from build123d import *

# Parameters (mm, degrees)
BOSS_EXTRUDE1_DEPTH = 1.5875
SKETCH3_W           = 9.525
SKETCH3_H           = 2.54
CUT_EXTRUDE1_DEPTH  = 29.598819744
SKETCH4_R           = 1.5875
BOSS_EXTRUDE2_DEPTH = 2.54
BOSS_EXTRUDE3_DEPTH = 1.778
SKETCH6_W           = 48.787
SKETCH6_H           = 0.4318
CUT_EXTRUDE2_DEPTH  = 19.05


with BuildPart() as part:
    # Sketch2 → Boss-Extrude1 (new body)
    with BuildSketch(Plane.XY):
        with BuildLine():
            Line((21.2185, 2.909935566), (21.2185, 11.9225))
            ThreePointArc((21.2185, 11.9225), (20.362958908, 13.987958908), (18.2975, 14.8435))
            Line((18.2975, 14.8435), (-18.2975, 14.8435))
            ThreePointArc((-18.2975, 14.8435), (-20.362958908, 13.987958908), (-21.2185, 11.9225))
            Line((-21.2185, 11.9225), (-21.2185, 2.909935566))
            ThreePointArc((-21.2185, 2.909935566), (-24.3935, 0), (-21.2185, -2.909935566))
            Line((-21.2185, -2.909935566), (-21.2185, -11.9225))
            ThreePointArc((-21.2185, -11.9225), (-20.362958908, -13.987958908), (-18.2975, -14.8435))
            Line((-18.2975, -14.8435), (18.2975, -14.8435))
            ThreePointArc((18.2975, -14.8435), (20.362958908, -13.987958908), (21.2185, -11.9225))
            Line((21.2185, -11.9225), (21.2185, -2.909935566))
            ThreePointArc((21.2185, -2.909935566), (24.3935, 0), (21.2185, 2.909935566))
        make_face()
    extrude(amount=BOSS_EXTRUDE1_DEPTH)

    # Sketch3 → Cut-Extrude1 (cut, through all)
    with BuildSketch(Plane.XY.offset(1.5875)):
        with Locations((0, -13.5735)):
            Rectangle(SKETCH3_W, SKETCH3_H)
        with Locations((0, 13.5735)):
            Rectangle(SKETCH3_W, SKETCH3_H)
    extrude(amount=-CUT_EXTRUDE1_DEPTH, mode=Mode.SUBTRACT)

    # Sketch4 → Boss-Extrude2 (add)
    with BuildSketch(Plane(origin=(0, 0, 0), x_dir=(-1, 0, 0), z_dir=(0, 0, -1))):
        with Locations(Location((-21.4725, 0, 0), (0, 0, 180))):
            Circle(SKETCH4_R)
        with Locations(Location((21.4725, 0, 0), (0, 0, 180))):
            Circle(SKETCH4_R)
    extrude(amount=BOSS_EXTRUDE2_DEPTH)

    # Sketch5 → Boss-Extrude3 (add)
    with BuildSketch(Plane(origin=(0, 0, 0), x_dir=(-1, 0, 0), z_dir=(0, 0, -1))):
        Polygon((-19.757999981, 9.854397583), (-16.165897533, 13.446500031), (-4.7625, 13.446500031), (-4.7625, 12.3035), (4.7625, 12.3035), (4.7625, 13.446500031), (16.229397533, 13.446500031), (19.821499981, 9.854397583), (19.821499981, -9.854397583), (16.229397533, -13.446500031), (4.7625, -13.446500031), (4.7625, -12.3035), (-4.7625, -12.3035), (-4.7625, -13.446500031), (-16.165897533, -13.446500031), (-19.757999981, -9.854397583), align=None)
    extrude(amount=BOSS_EXTRUDE3_DEPTH)

    # Sketch6 → Cut-Extrude2 (cut, symmetric)
    with BuildSketch(Plane(origin=(0, 0, 0), x_dir=(1, 0, 0), z_dir=(0, 1, 0))):
        with Locations((0, -1.3716)):
            Rectangle(SKETCH6_W, SKETCH6_H)
    extrude(amount=CUT_EXTRUDE2_DEPTH, both=True, mode=Mode.SUBTRACT)


solid = part.part
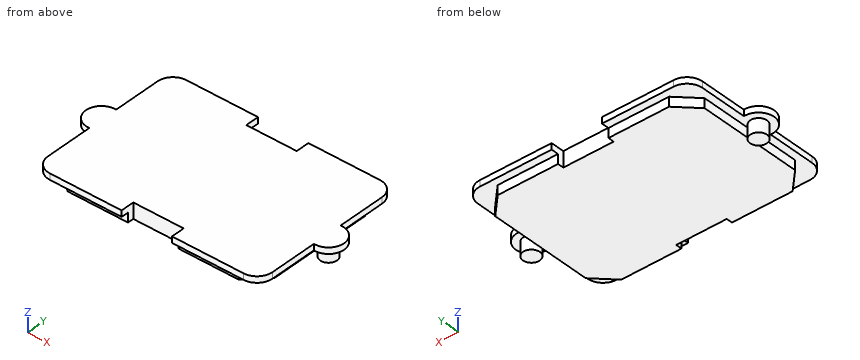
Geometry check sheet. Reference: the model listing, model coordinates, mm. Give positions to 0.01 mm unless a question says otherwise; leave off trailing zeros. Loops run counter-clockwise (first coordinate to the right, second up) from the corner with the lowest first, then second, coordinate; pieces in that order, holes last.
(1) Section check C-C on x = 8. Record the cut outline in (y, z), then the cut area to 3 significant figures.
From the geometry:
outline: (-14.84, 0) - (-13.45, 0) - (-13.45, -1.78) - (13.45, -1.78) - (13.45, 0) - (14.84, 0) - (14.84, 1.16) - (-14.84, 1.16) - close
area: 82.1 mm2
(2) Depth check by flat-ended pin: pin 1 Ø0.8 at (y, z) = (-13.5, 0) entering from +X; pin 2 Ø0.9 at (x, z) = (11, -1) entering from -Y; pin 3 Ø0.8 at (y, z) = (14, -1) entering from +X; pin 4 Ø10 at (x, y) = (14, 2) entering from -Z. Enter the tip coordinate at first touch or a pass-through.
From the geometry:
pin 1: stops at x = 20.97
pin 2: stops at y = -13.45
pin 3: passes through
pin 4: stops at z = -1.78
(3) Section check B-B on z = -1.1. Record the cut outline in (x, y) (1 decimal), then the cut area to 3 significant figures.
From the geometry:
outline: circle Ø3.2 at (-21.5, 0); (-19.8, -9.9) - (-16.2, -13.4) - (-4.8, -13.4) - (-4.8, -12.3) - (4.8, -12.3) - (4.8, -13.4) - (16.2, -13.4) - (19.8, -9.9) - (19.8, 9.9) - (16.2, 13.4) - (4.8, 13.4) - (4.8, 12.3) - (-4.8, 12.3) - (-4.8, 13.4) - (-16.2, 13.4) - (-19.8, 9.9) - close; circle Ø3.2 at (21.5, 0)
area: 1,030 mm2
(4) Thickness scan on L1, parallel to X at y = 1.25, z = -0.75; L2, parallel to Z at x = -9.5, y = -1.5; L3, parallel to X at y = -3.75, z = -1.4. Record the ranges inside material, lowest first.
From the geometry:
L1: x = -22.45 to -20.49, -19.82 to 19.76, 20.49 to 22.45
L2: z = -1.78 to 1.16
L3: x = -19.82 to 19.76
(5) Section check D-D on y = 7.5. Record the cut outline in (x, z), then the cut area to 3 significant figures.
From the geometry:
outline: (-21.22, 0) - (-19.82, 0) - (-19.82, -1.78) - (19.76, -1.78) - (19.76, 0) - (21.22, 0) - (21.22, 1.16) - (-21.22, 1.16) - close
area: 119 mm2
